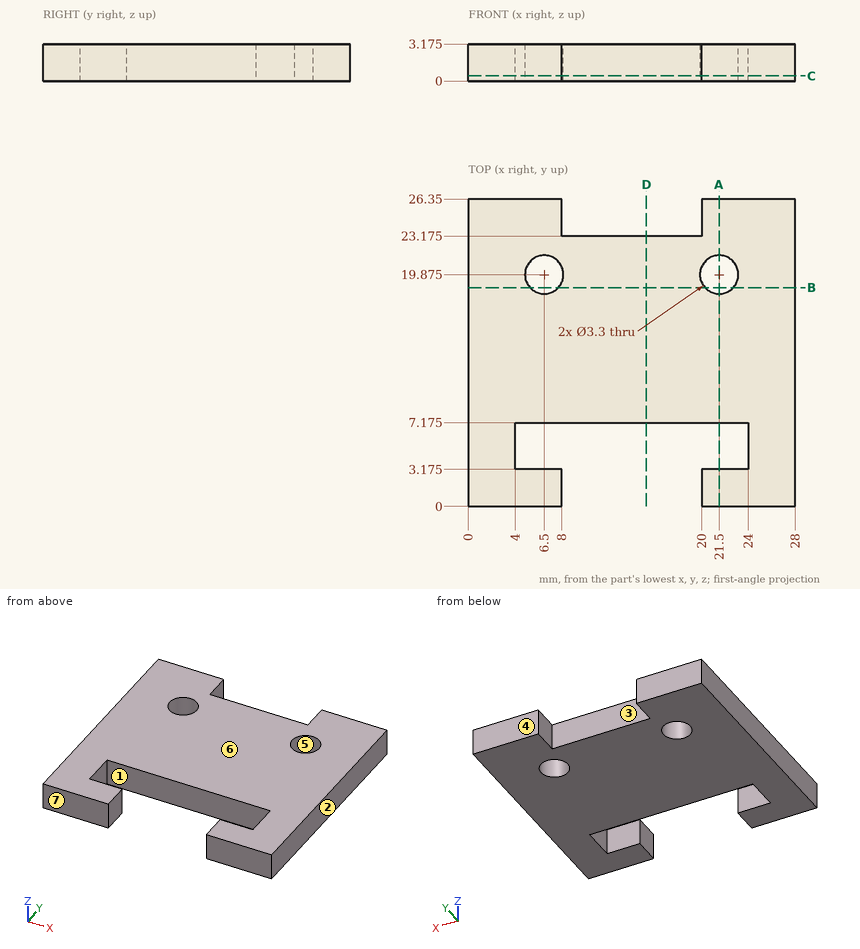
Source: three-view drawing plus pictorial views. Frame: mm from the lowest corner of the part. A direction names the side the tool comes from. Round coordinates to 2 decimals unless told otherwise and drop trailing zeros. Order: outer loops, then holes, each group sorted by start corner. A loop starts at its lowest first (then second) coordinate and runs counter-clockwise, first axis right, second up. Notation, with made-up numbers: (66, 44) -> (90, 44) arc R14 ccw to (90, 56) -> close; hole circle Ø8 at (-26, 1). An arc over 180 degrees is marked (long way). Use CSV: the item, a comma, the result in double quotes. Start each with the question number.
1) Section A-A (x = 21.5). Return the cut outline in (y, z) (3 decimals), and give its area (3 significant figures).
2) Material intervals for line 1 along X through (y, z) = (19.75, 3); line 2 along Y through (x, z) = (6.5, 1.7) (3 decimals); line 3 along X through (y, z) = (3.75, 1.8), sorted ascending. Write a range as from..to.
3) Draft query along Y for the marked faces 4, 5, 6 and 7. Return one class per face: +Y half, -Y half, draft (parallel to the pull), parting line (faces both ways), or undercut.
4) Section D-D (x = 15.25). Return the cut outline in (y, z) (3 decimals), and give its area (3 significant figures).
5) Section C-C (z = 0.45). Return the cut outline in (x, y) (3 decimals).
6) Section B-B (y = 18.75). Return the cut outline in (x, z) (3 decimals).
7) Set-up query: the marked faces 1, 2 and 3. Return all of +Z, -Z, +X, -X, +Y, -Y with unobstructed straight access to the full face (end or side cutting, diameter ignored); none if empty.
8) First-contact query: pin 1 Ø2 at (x, y) = (21.5, 19.875) entering from -Z; pin 2 Ø1.6 at (x, z) = (14.5, 2) entering from +Y (3 decimals). Flat tips, straight axial feed; report the tip coordinate or a pass-through.
Returned:
1,outline,"(0, 0) -> (3.175, 0) -> (3.175, 3.175) -> (0, 3.175) -> close; (7.175, 0) -> (18.225, 0) -> (18.225, 3.175) -> (7.175, 3.175) -> close; (21.525, 0) -> (26.35, 0) -> (26.35, 3.175) -> (21.525, 3.175) -> close"
1,area,"60.5 mm²"
2,line 1,"x = 0..4.85, 8.15..19.85, 23.15..28"
2,line 2,"y = 0..3.175, 7.175..18.225, 21.525..26.35"
2,line 3,"x = 0..4, 24..28"
3,face 4,"+Y half"
3,face 5,"undercut"
3,face 6,"draft"
3,face 7,"-Y half"
4,outline,"(7.175, 0) -> (23.175, 0) -> (23.175, 3.175) -> (7.175, 3.175) -> close"
4,area,"50.8 mm²"
5,outline,"(0, 0) -> (8, 0) -> (8, 3.175) -> (4, 3.175) -> (4, 7.175) -> (24, 7.175) -> (24, 3.175) -> (20, 3.175) -> (20, 0) -> (28, 0) -> (28, 26.35) -> (20, 26.35) -> (20, 23.175) -> (8, 23.175) -> (8, 26.35) -> (0, 26.35) -> close; hole circle Ø3.3 at (6.5, 19.875); hole circle Ø3.3 at (21.5, 19.875)"
6,outline,"(0, 0) -> (5.293, 0) -> (5.293, 3.175) -> (0, 3.175) -> close; (7.707, 0) -> (20.293, 0) -> (20.293, 3.175) -> (7.707, 3.175) -> close; (22.707, 0) -> (28, 0) -> (28, 3.175) -> (22.707, 3.175) -> close"
7,face 1,"+Z, -Z"
7,face 2,"+Z, -Z, +X, +Y, -Y"
7,face 3,"+Z, -Z, +Y"
8,pin 1,"passes through"
8,pin 2,"stops at y = 23.175"
